```python
from build123d import *

# Parameters (mm, degrees)
ESBO_O1_W                = 12.4
ESBO_O1_H                = 25
RESSALTO_EXTRUS_O1_DEPTH = 3
FILETE1_R                = 2


with BuildPart() as part:
    # Esboço1 → Ressalto-extrusão1 (new body)
    with BuildSketch(Plane(origin=(0, 0, 0), x_dir=(0, 0, -1), z_dir=(1, 0, 0))):
        with BuildLine():
            Line((-8, 19), (8, 19))
            Line((8, 19), (8, -19))
            Line((8, -19), (1.25078293, -35.963499669))
            ThreePointArc((1.25078293, -35.963499669), (0.883014852, -36.421369201), (0.321624406, -36.593818135))
            Line((0.321624406, -36.593818135), (-0.321624406, -36.593818135))
            ThreePointArc((-0.321624406, -36.593818135), (-0.883014852, -36.421369201), (-1.25078293, -35.963499669))
            Line((-1.25078293, -35.963499669), (-8, -19))
            Line((-8, -19), (-8, 19))
        make_face()
        Rectangle(ESBO_O1_W, ESBO_O1_H, mode=Mode.SUBTRACT)
    extrude(amount=RESSALTO_EXTRUS_O1_DEPTH)

    # Filete1
    filete1_edges = [part.edges().sort_by_distance(p)[0] for p in [
        (1.5, 19, 8),
        (1.5, 19, -8),
    ]]
    fillet(filete1_edges, radius=FILETE1_R)


solid = part.part
```
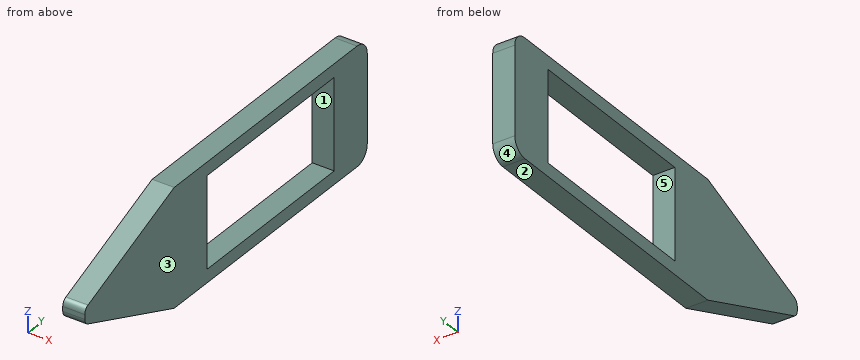
Geometry check sheet. Reference: the model listing, model coordinates, mm. Face numbers are marked on the shaded views. A direction names the side the tool comes from. Round coordinates to 2 decimals unless told otherwise and drop trailing zeros. Write each loop counter-clockwise with the first axis right and the second up, starting at its lowest first coordinate (ties: lowest second). Pieces come first, ordered by that corner, then holes. Notation, with made-up numbers: (-5, -15) -> (46, -15) arc R10 cw to (46, 2) -> close; hole circle Ø2 at (-17, 20). An arc over 180 degrees is marked (long way). Put each result on its own line as item: value.
1) Thickness scan on probe 1 along Z at (x, y) = (0.8, -9.5); probe 2 along Y at (x, z) = (2.6, -0.25); probe 3 along Y at (x, z) = (1.7, 1). Record the ranges inside material, lowest first. Write a range as from..to.
Recorded:
probe 1: z = -8..-6.2, 6.2..8
probe 2: y = -36.59..-12.5, 12.5..19
probe 3: y = -36.33..-12.5, 12.5..19
2) Cross-section at D-D, the plane y = -23. Enter the section's corners in (x, z).
Recorded:
outline: (0, -6.41) -> (3, -6.41) -> (3, 6.41) -> (0, 6.41) -> close
3) Cross-section at C-C, the plane z = -5. Enter the section's corners in (x, y), plus the area to 3 significant figures.
Recorded:
outline: (0, -26.54) -> (3, -26.54) -> (3, -12.5) -> (0, -12.5) -> close; (0, 12.5) -> (3, 12.5) -> (3, 19) -> (0, 19) -> close
area: 61.6 mm2
4) Cross-section at A-A, the plane y = -3. Enter the section's corners in (x, z), plus the area to 3 significant figures.
Recorded:
outline: (0, -8) -> (3, -8) -> (3, -6.2) -> (0, -6.2) -> close; (0, 6.2) -> (3, 6.2) -> (3, 8) -> (0, 8) -> close
area: 10.8 mm2
5) Cross-section at B-B, the plane x = 1.3. Enter the section's corners in (y, z), plus the area to 3 significant figures.
Recorded:
outline: (-36.59, -0.32) arc R1 ccw to (-35.96, -1.25) -> (-19, -8) -> (17, -8) arc R2 ccw to (19, -6) -> (19, 6) arc R2 ccw to (17, 8) -> (-19, 8) -> (-35.96, 1.25) arc R1 ccw to (-36.59, 0.32) -> close; hole (-12.5, -6.2) -> (12.5, -6.2) -> (12.5, 6.2) -> (-12.5, 6.2) -> close
area: 454 mm2
6) Access from +Z, -Z, +X, -X, +Y, -Y to the whole of each face (thin tool, end or side, straight path). Record for the marked faces 4 and 5.
Recorded:
face 4: -Z, +X, -X, +Y
face 5: +X, -X
7) Release check for a two-part mould opening along Z. For the marked faces 1, 2 and 3 record: pulls with the +Z half, pulls with the -Z half, needs draft (parallel to the pull), parting line crosses it, or undercut.
Recorded:
face 1: undercut
face 2: pulls with the -Z half
face 3: needs draft
